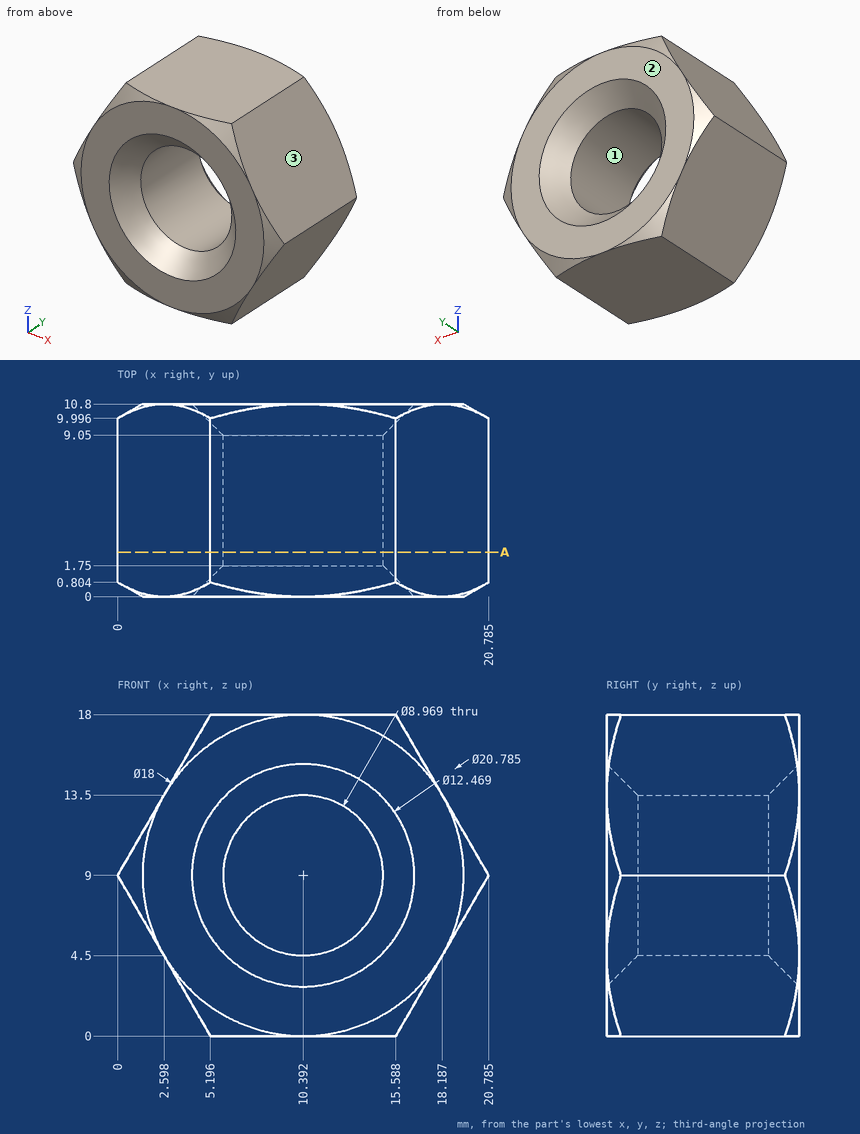
Drawing for the job (mm, zero at the part's lowest x, y, z). Round coordinates to 2 decimals unless told otherwise and drop trailing zeros. Loops run counter-clockwise (first coordinate to the right, second up) from the corner with the lowest first, then second, coordinate; pieces in that order, holes last. Notation, with made-up numbers: M 19.25,-14 L 55.25,-14 A16 ccw 55.25,14 Z; hole C 77.5,-30.75 d2. An arc over 180 degrees is marked long. Use a Markdown table: item, result. Add a question column.
(1) Flat gauge pins, fed straight in: pin 1 (3 mm diameter, centred on y = 6.5, z = 7, fed in from -X); pin 2 (1.5 mm diameter, centred on x = 7.5, z = 6.5, fed in from -Y); pin 3 (1.5 mm diameter, centred on y = 1.5, z = 4.5, fed in from +X). Where does each tip first touch, or does it go through?
(2) Drill centre lines: line 1 (Z direction, x = 11.75, y = 10.25); line 2 (Z direction, x = 11, y = 8.75); line 3 (X direction, y = 4.5, z = 5) (1 decimal). Where is each one in solid material? Low to high.
(3) Pull direction Z, two halves, no side cores. Call the marked faces 1, 2 and 3: +Z half, -Z half, draft (parallel to the pull), parting line (faces both ways), or undercut.
(4) Cut at A-A (y = 2.5). Give the cut face in (x, z) (1 decimal).
Geometry says:
| question | item | result |
|---|---|---|
| 1 | pin 1 | stops at x = 0.29 |
| 1 | pin 2 | stops at y = 1.66 |
| 1 | pin 3 | stops at x = 18.62 |
| 2 | line 1 | z = 0 to 3.48, 14.52 to 18 |
| 2 | line 2 | z = 0 to 4.56, 13.44 to 18 |
| 2 | line 3 | x = 2.3 to 8.4, 12.4 to 18.5 |
| 3 | face 1 | undercut |
| 3 | face 2 | draft |
| 3 | face 3 | +Z half |
| 4 | outline | M 0,9 L 5.2,0 L 15.6,0 L 20.8,9 L 15.6,18 L 5.2,18 Z; hole C 10.4,9 d9 |
